Verification items for this drawing (mm, ordinates from the low corner). A direction names the side the tool comes from. Coordinates: 2 decimals unless noted, no trailing zeros. Order: outer loops, then holes, each group sorted by start corner. A loop starts at its lowest first (then second) coordinate and runs counter-clockwise, first axis right, second up. Notation, with made-up numbers: (83, -21) - (125, -21) arc R20 cw to (125, -2) - close; hole circle Ø4 at (-33.75, 49.5). An arc over 180 degrees is marked (long way). Use CSV: the item, a comma, the result in double quotes. Start each with the question number.
1) Sectioned sample at A-A, the plane x = 7. Record the cut outline in (y, z).
2) Sectioned sample at B-B, the plane y = 4.5. Record the cut outline in (x, z), and give its area (3 significant figures).
3) Thickness scan on probe 1 along X at (y, z) = (7, 2); probe 2 along X at (y, z) = (11.25, 6.75). Record the ranges inside material, lowest first. Write a range as [from, to].
4) Sectioned sample at C-C, the plane z = 7. Record the cut outline in (x, y), and give its area (3 significant figures).
5) Tool access check on the marked faces 4 and 5. Record the directions out of +Z, -Z, +X, -X, +Y, -Y that give a thin tool (end or side, any length) a straight path to the whole face; none if there is none.
6) Draft check along Y on the marked faces 1, 2 and 3. Enter one of: released by +Y, released by -Y, zero draft, split by the parting line, or undercut.
7) Sectioned sample at D-D, the plane z = 4. Record the cut outline in (x, y).
8) Depth check by flat-ended pin: P1, Ø1.5, axis at x = 1.5, z = 4, coming from the +Y side; P2, Ø3, axis at y = 9, z = 5, coming from the -X side; P3, Ø1, axis at x = 4.5, y = 1.5, coming from the +Z side; P4, Ø6, axis at y = 9, z = 4, coming from the +X side. Enter the tip coordinate at first touch or a pass-through.
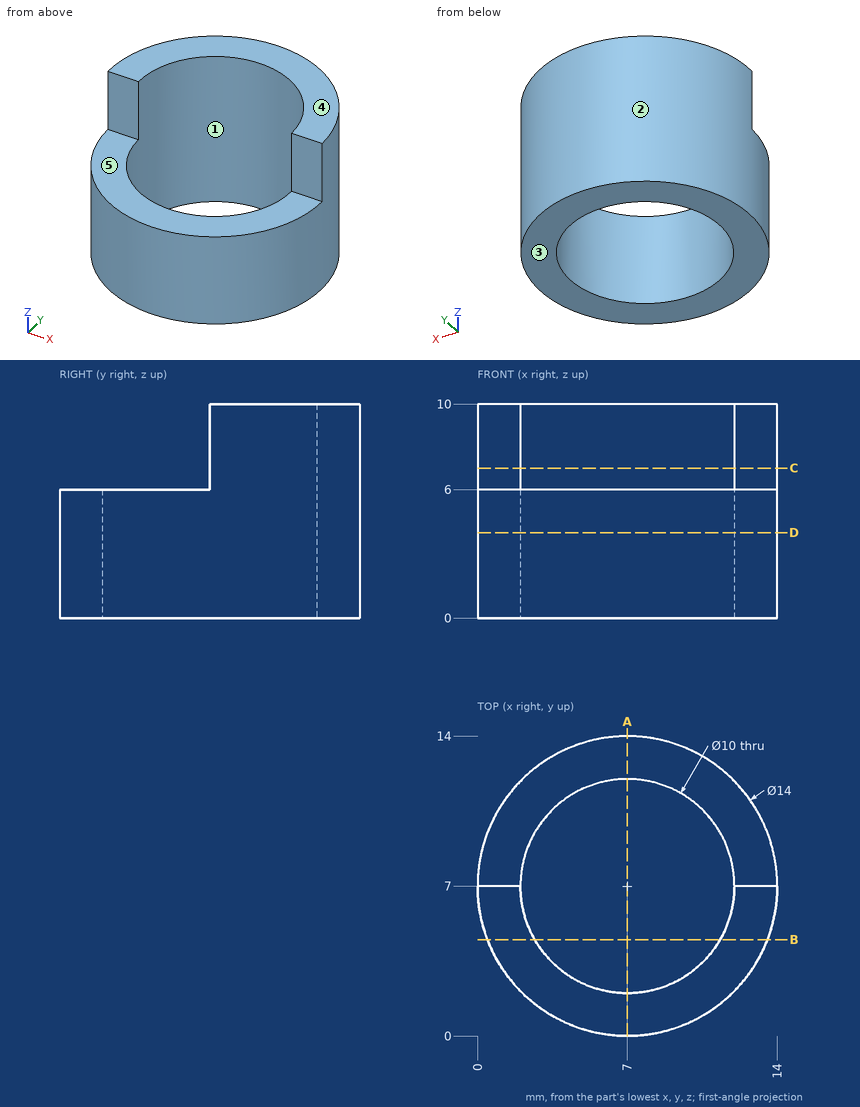
Evaluation:
1,outline,"(0, 0) - (2, 0) - (2, 6) - (0, 6) - close; (12, 0) - (14, 0) - (14, 10) - (12, 10) - close"
2,outline,"(0.46, 0) - (2.67, 0) - (2.67, 6) - (0.46, 6) - close; (11.33, 0) - (13.54, 0) - (13.54, 6) - (11.33, 6) - close"
2,area,"26.5 mm²"
3,probe 1,"[0, 2], [12, 14]"
3,probe 2,"[1.44, 4.37], [9.63, 12.56]"
4,outline,"(0, 7) - (2, 7) arc R5 cw to (12, 7) - (14, 7) arc R7 ccw to start"
4,area,"37.7 mm²"
5,face 4,"+Z, +X, -X, +Y, -Y"
5,face 5,"+Z, +X, -X, -Y"
6,face 1,"undercut"
6,face 2,"split by the parting line"
6,face 3,"zero draft"
7,outline,"circle Ø14 at (7, 7); hole circle Ø10 at (7, 7)"
8,P1,"y = 12.14"
8,P2,"x = 0.02"
8,P3,"z = 6"
8,P4,"x = 14"
